Check sheet for the drawn part. Datum: minimum x, y, z corner. Units: mm. Round coordinates to 2 decimals unless told otherwise and drop trailing zeros. Write each loop counter-clockwise with the first axis right and the second up, starting at its lowest first coordinate (ties: lowest second). Pieces come first, ordered by that corner, then holes. Notation, with made-up numbers: (14, 24) - (43, 24) arc R17 ccw to (43, 54) - close; hole circle Ø11 at (-2.5, -10.75). An arc over 180 degrees is marked (long way). Answer as a JSON object with one key per item and string values.
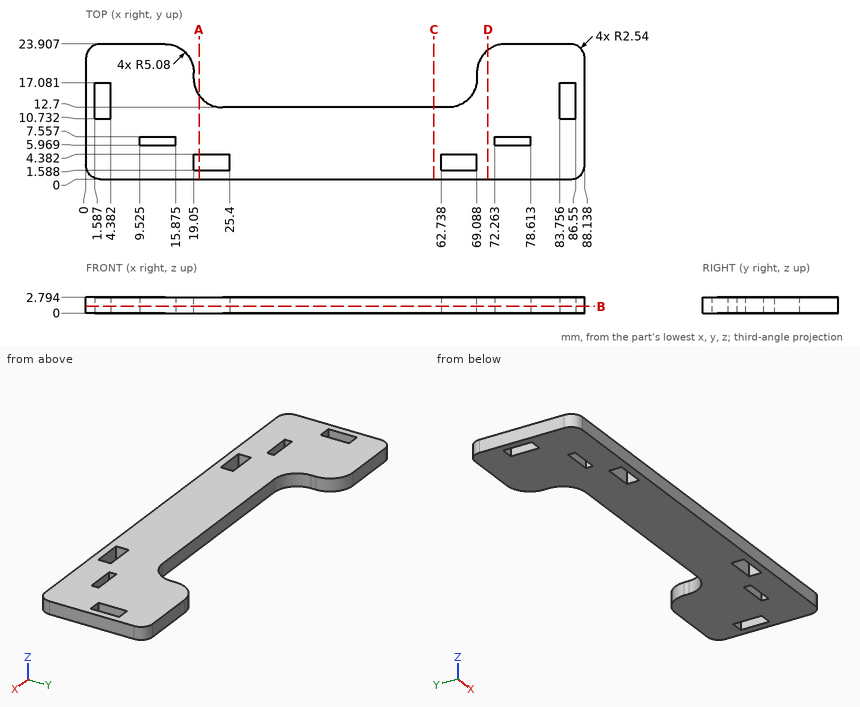
1. Cross-section at B-B (z = 1.2). Count the separate pieces of the cut face and the enclosed holes in it, plus the area to 3 significant figures.
Completed:
{"separate pieces": "1", "enclosed holes": "6", "area": "1,450 mm^2"}
2. Cross-section at A-A (x = 20). Record the boundary of the cut face in (y, z) (1 decimal), plus the area to 3 significant figures.
Completed:
{"outline": "(0, 0) - (1.6, 0) - (1.6, 2.8) - (0, 2.8) - close; (4.4, 0) - (14.8, 0) - (14.8, 2.8) - (4.4, 2.8) - close", "area": "33.6 mm^2"}
3. Cross-section at D-D (x = 71). Record the boundary of the cut face in (y, z) (1 decimal).
Completed:
{"outline": "(0, 0) - (22.8, 0) - (22.8, 2.8) - (0, 2.8) - close"}
4. Go/stop test with a flat-tipped pin: pin 1 (0.8 mm diameter, centred on y = 3.5, z = 1, fed in from -X). Record where the tip stops, or that it passes through.
Completed:
{"pin 1": "stops at x = 0"}
5. Cross-section at C-C (x = 61.5). Record the boundary of the cut face in (y, z) (1 decimal), plus the area to 3 significant figures.
Completed:
{"outline": "(0, 0) - (12.7, 0) - (12.7, 2.8) - (0, 2.8) - close", "area": "35.5 mm^2"}
6. Material ranges on probe 1 along X at (y, z) = (3.75, 0.2); probe 2 along X at (y, z) = (12.5, 1.8); probe 3 along Y at (x, z) = (63, 1.3), recorded low to high. Write a range as from..to.
Completed:
{"probe 1": "x = 0..19.05, 25.4..62.74, 69.09..88.14", "probe 2": "x = 0..1.59, 4.38..83.76, 86.55..88.14", "probe 3": "y = 0..1.59, 4.38..12.7"}
